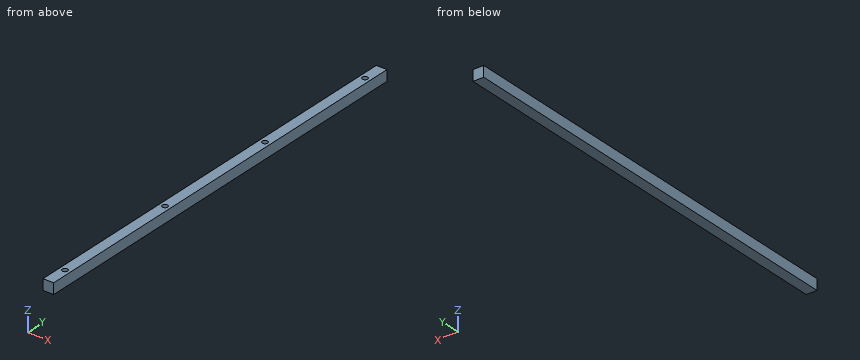
from build123d import *

# Parameters (mm, degrees)
F0_W     = 50
F0_H     = 50
F1_DEPTH = 2000
F2_R     = 12.5
F3_DEPTH = 25


with BuildPart() as f1:
    # F0 (on Front) → F1 (new body)
    with BuildSketch(Plane.XZ):
        with Locations((25, 25)):
            Rectangle(F0_W, F0_H)
    extrude(amount=-F1_DEPTH)

    # F2 (on face) → F3 (cut)
    with BuildSketch(Plane.XY.offset(50)):
        with Locations((25, 100)):
            Circle(F2_R)
        with Locations((25, 1900)):
            Circle(F2_R)
        with Locations((25, 1300)):
            Circle(F2_R)
        with Locations((25, 700)):
            Circle(F2_R)
    extrude(amount=-F3_DEPTH, mode=Mode.SUBTRACT)


solid = f1.part
Work out the finished part from the listing and answer in its coordinate system (mm). Give positions to 0.01 mm unless a question says otherwise; leave off trailing zeros. Write each loop counter-clockwise with the first axis right and the second up, starting at its lowest first coordinate (ties: lowest second). Pieces come first, ordered by that corner, then holes. Notation, with made-up numbers: (19.5, 34.25) - (45.5, 34.25) arc R35 ccw to (45.5, 67.25) - close; hole circle Ø5 at (17.25, 62.25). An arc over 180 degrees is marked (long way). One line per item, written item: value. Start each with the question number.
1. Given pin 1 (7.5 mm diameter, centred on x = 28, y = 1300, fed in from +Z), flat-ended and moving along its own axis, determine where the tip first touches the part or whether it passes through.
2. Consider probe 1 along Y at (x, z) = (25, 30); probe 2 along X at (y, z) = (1900, 42.5); probe 3 along Y at (x, z) = (20, 27). Determine where each line is inside the solid, lowest interval first.
3. Find section B-B (x = 25). Write down the section's boundary in (y, z).
4. Find section A-A (z = 41). Write down the section's boundary in (x, y).
Geometry results:
1. pin 1: z = 25
2. probe 1: 0 to 87.5, 112.5 to 687.5, 712.5 to 1287.5, 1312.5 to 1887.5, 1912.5 to 2000
2. probe 2: 0 to 12.5, 37.5 to 50
2. probe 3: 0 to 88.54, 111.46 to 688.54, 711.46 to 1288.54, 1311.46 to 1888.54, 1911.46 to 2000
3. outline: (0, 0) - (2000, 0) - (2000, 50) - (1912.5, 50) - (1912.5, 25) - (1887.5, 25) - (1887.5, 50) - (1312.5, 50) - (1312.5, 25) - (1287.5, 25) - (1287.5, 50) - (712.5, 50) - (712.5, 25) - (687.5, 25) - (687.5, 50) - (112.5, 50) - (112.5, 25) - (87.5, 25) - (87.5, 50) - (0, 50) - close
4. outline: (0, 0) - (50, 0) - (50, 2000) - (0, 2000) - close; hole circle Ø25 at (25, 100); hole circle Ø25 at (25, 700); hole circle Ø25 at (25, 1300); hole circle Ø25 at (25, 1900)
